Build history of the part. All positions in model axes, mm. A direction names the side the tool comes from. Give positions to 0.01 mm unless a question says otherwise; leave off trailing zeros. Loops run counter-clockwise (first coordinate to the right, second up) from the corner with the lowest first, then second, coordinate; pieces in that order, holes last. Notation, with made-up numbers: (-34, 47) -> (-26, 47) arc R32 cw to (-26, 74) -> close; hole circle Ø3 at (62, 68.25). An arc over 180 degrees is marked (long way). Answer as a JSON object with one key per item and string values. Group by question number.
Q1. Wall check: probe 1 along X at (y, z) = (-1.75, -51); probe 2 along X at (y, z) = (-4.5, -2); probe 3 along X at (y, z) = (-1, 49). Give the ranges that are in metal, low to high. Write a range as from..to.
Q2. Tool access for faces 1 (the flat face through (-105, -3, -1)), 2 (the flat face through (78.1, -3, 2)): list every direction of +Z, -Z, +X, -X, +Y, -Y with a clear straight run to the whole face (end or side of a thin tool).
Q3. Two-plate mould, pull along X, no slides. Class faces 3 (the cylindrical face through (50, -3.1, 4.1)), 4 (the flat face through (22, 0, 1)), 5 (the cylindrical face through (9.69, -3.13, -16.13)), 6 (the flat face through (105, -3, -1)): pulls with the +X half, pulls with the -X half, needs draft (parallel to the pull), parting line crosses it, or undercut.
Q4. Band-saw the part on D-D, the plane x = 68. Write the cut outline in (y, z), plus the area to 3 significant figures.
Q5. Band-saw the part on B-B, the plane z = -13.5. Write the cut outline in (x, y).
Q6. Drop a flat-ended pin along its axis: pin 1 (8.5 mm diameter, centred on x = 45, z = 2.5, fed in from -Y). Give the stop position or say it passes through.
Q7. Band-saw the part on A-A, the plane x = 0. Write the cut outline in (y, z), plus the area to 3 significant figures.
Q8. Band-saw the part on C-C, the plane y = -5.25. Count the separate pieces of the cut face and the enclosed holes in it, plus the area to 3 significant figures.
from build123d import *

# Parameters (mm, degrees)
F0_W     = 209.999986
F0_H     = 135.000009
F0_R     = 4.499991
F0_R_2   = 2.116988
F0_R_3   = 5.250002
F0_W_2   = 3.199994
F0_H_2   = 25.2
F0_R_4   = 21.000009
F0_W_3   = 3.199993
F1_DEPTH = 6.35


with BuildPart() as f1:
    # F0 (on Front) → F1 (new body)
    with BuildSketch(Plane.XZ):
        with Locations((0, -1.3e-05)):
            Rectangle(F0_W, F0_H)
        with Locations((-89.999998, -52.499997)):
            Circle(F0_R, mode=Mode.SUBTRACT)
        with Locations((-45.000012, -54.500018)):
            Circle(F0_R_2, mode=Mode.SUBTRACT)
        with Locations((45.000012, -54.500018)):
            Circle(F0_R_2, mode=Mode.SUBTRACT)
        with Locations((66.999993, -52.908505)):
            Circle(F0_R_3, mode=Mode.SUBTRACT)
        with Locations((89.999998, -52.499997)):
            Circle(F0_R, mode=Mode.SUBTRACT)
        with Locations((-65.599996, 2.399995)):
            Rectangle(F0_W_2, F0_H_2, mode=Mode.SUBTRACT)
        with Locations((-44.999986, 2.499995)):
            Circle(F0_R_3, mode=Mode.SUBTRACT)
        with Locations((0, 2.499995)):
            Circle(F0_R_4, mode=Mode.SUBTRACT)
        with Locations((-89.999998, 52.499997)):
            Circle(F0_R, mode=Mode.SUBTRACT)
        with Locations((45.000012, 2.499995)):
            Circle(F0_R_3, mode=Mode.SUBTRACT)
        with Locations((76.5, 2.499995)):
            Rectangle(F0_W_3, F0_H_2, mode=Mode.SUBTRACT)
        with Locations((66.999993, 52.499997)):
            Circle(F0_R_3, mode=Mode.SUBTRACT)
        with Locations((89.999998, 52.499997)):
            Circle(F0_R, mode=Mode.SUBTRACT)
    extrude(amount=F1_DEPTH)


solid = f1.part
Worked answers:
{
 "1": {"probe 1": "-105..-94.24, -85.76..62.11, 71.89..85.76, 94.24..105", "probe 2": "-105..-67.2, -64..-47.7, -42.3..-20.51, 20.51..42.3, 47.7..74.9, 78.1..105", "probe 3": "-105..-92.83, -87.17..63.09, 70.91..87.17, 92.83..105"},
 "2": {"face 1": "+Z, -Z, -X, +Y, -Y", "face 2": "+Y, -Y"},
 "3": {"face 3": "undercut", "face 4": "needs draft", "face 5": "undercut", "face 6": "pulls with the +X half"},
 "4": {"outline": "(-6.35, -67.5) -> (0, -67.5) -> (0, -58.06) -> (-6.35, -58.06) -> close; (-6.35, -47.75) -> (0, -47.75) -> (0, 47.35) -> (-6.35, 47.35) -> close; (-6.35, 57.65) -> (0, 57.65) -> (0, 67.5) -> (-6.35, 67.5) -> close", "area": "726 mm2"},
 "5": {"outline": "(-105, -6.35) -> (-13.6, -6.35) -> (-13.6, 0) -> (-105, 0) -> close; (13.6, -6.35) -> (105, -6.35) -> (105, 0) -> (13.6, 0) -> close"},
 "6": {"pin 1": "through"},
 "7": {"outline": "(-6.35, -67.5) -> (0, -67.5) -> (0, -18.5) -> (-6.35, -18.5) -> close; (-6.35, 23.5) -> (0, 23.5) -> (0, 67.5) -> (-6.35, 67.5) -> close", "area": "591 mm2"},
 "8": {"separate pieces": "1", "enclosed holes": "13", "area": "26,200 mm2"}
}
